Verification items for the finished model (mm, model axes). Coordinates: 2 decimals unless noted, no trailing zeros. Loops run counter-clockwise (first coordinate to the right, second up) from the corner with the lowest first, then second, coordinate; pieces in that order, holes last. Notation, with made-up numbers: (-31.75, 56.5) -> (-14.75, 56.5) arc R21 ccw to (-14.75, 71.5) -> close; hole circle Ø6 at (0, 10). An arc over 180 degrees is marked (long way). Write item = value, one per line.
```python
from build123d import *

# Parameters (mm, degrees)
F1_DEPTH = 3.048


with BuildPart() as f1:
    # F0 (on Front) → F1 (new body)
    with BuildSketch(Plane.XZ):
        with BuildLine():
            Line((9.525, 0), (0, 0))
            Line((0, 0), (0, 9.525))
            ThreePointArc((0, 9.525), (-5.473729162, 7.7951211704), (-8.95924033, 3.2338270994))
            ThreePointArc((-8.95924033, 3.2338270994), (-6.4472498387, -7.0113190283), (3.9721601425, -8.657226392))
            ThreePointArc((3.9721601425, -8.657226392), (8.0174949441, -5.1425090978), (9.525, 0))
        make_face()
        with BuildLine():
            Line((0, 9.525), (0, 0))
            Line((0, 0), (9.525, 0))
            ThreePointArc((9.525, 0), (8.5520017953, 4.1939110974), (5.8317946892, 7.5309890255))
            ThreePointArc((5.8317946892, 7.5309890255), (3.0816354856, 9.0127214388), (0, 9.525))
        make_face()
        with BuildLine():
            ThreePointArc((-8.95924033, 3.2338270994), (-5.473729162, 7.7951211704), (0, 9.525))
            Line((0, 9.525), (0, 47.625))
            ThreePointArc((0, 47.625), (-8.2836905365, 49.957618522), (-14.1330264303, 56.2699800194))
            Line((-14.1330264303, 56.2699800194), (-8.95924033, 3.2338270994))
        make_face()
        with BuildLine():
            Line((0, 47.625), (0, 9.525))
            ThreePointArc((0, 9.525), (3.0816354856, 9.0127214388), (5.8317946892, 7.5309890255))
            Line((5.8317946892, 7.5309890255), (14.4691487973, 56.9685868235))
            ThreePointArc((14.4691487973, 56.9685868235), (8.6118941245, 50.1639246932), (0, 47.625))
        make_face()
        with BuildLine():
            Line((36.5125, 0), (9.525, 0))
            ThreePointArc((9.525, 0), (8.0174949441, -5.1425090978), (3.9721601425, -8.657226392))
            Line((3.9721601425, -8.657226392), (40.3929904428, -6.8223588078))
            ThreePointArc((40.3929904428, -6.8223588078), (37.5504920607, -3.9243721084), (36.5125, 0))
        make_face()
        with BuildLine():
            ThreePointArc((5.8317946892, 7.5309890255), (8.5520017953, 4.1939110974), (9.525, 0))
            Line((9.525, 0), (36.5125, 0))
            ThreePointArc((36.5125, 0), (38.8078464582, 5.5830108061), (44.366360702, 7.9370593243))
            Line((44.366360702, 7.9370593243), (5.8317946892, 7.5309890255))
        make_face()
        with BuildLine():
            ThreePointArc((-14.1330264303, 56.2699800194), (-8.2836905365, 49.957618522), (0, 47.625))
            Line((0, 47.625), (0, 63.5))
            Line((0, 63.5), (0, 79.375))
            ThreePointArc((0, 79.375), (-10.4834895471, 75.4210767935), (-15.7448168762, 65.528883076))
            ThreePointArc((-15.7448168762, 65.528883076), (-15.6397954467, 60.7774233922), (-14.1330264303, 56.2699800194))
        make_face()
        with BuildLine():
            Line((0, 63.5), (0, 47.625))
            ThreePointArc((0, 47.625), (8.6118941245, 50.1639246932), (14.4691487973, 56.9685868235))
            ThreePointArc((14.4691487973, 56.9685868235), (15.5195580181, 60.1594994505), (15.875, 63.5))
            ThreePointArc((15.875, 63.5), (15.5195580181, 66.8405005495), (14.4691487973, 70.0314131765))
            ThreePointArc((14.4691487973, 70.0314131765), (8.6118941245, 76.8360753068), (0, 79.375))
            Line((0, 79.375), (0, 63.5))
        make_face()
        with BuildLine():
            ThreePointArc((44.366360702, 7.9370593243), (38.8078464582, 5.5830108061), (36.5125, 0))
            ThreePointArc((36.5125, 0), (37.5504920607, -3.9243721084), (40.3929904428, -6.8223588078))
            ThreePointArc((40.3929904428, -6.8223588078), (48.3743721084, -6.8995079393), (52.3875, 0))
            ThreePointArc((52.3875, 0), (50.0330108061, 5.6421535418), (44.366360702, 7.9370593243))
        make_face()
        with BuildLine():
            Line((0, 104.775), (0, 79.375))
            ThreePointArc((0, 79.375), (8.6118941245, 76.8360753068), (14.4691487973, 70.0314131765))
            Line((14.4691487973, 70.0314131765), (9.5153598494, 113.8715703832))
            ThreePointArc((9.5153598494, 113.8715703832), (6.581976637, 107.4150011946), (0, 104.775))
        make_face()
        with BuildLine():
            ThreePointArc((-15.7448168762, 65.528883076), (-10.4834895471, 75.4210767935), (0, 79.375))
            Line((0, 79.375), (0, 104.775))
            ThreePointArc((0, 104.775), (-6.581976637, 107.4150011946), (-9.5153598494, 113.8715703832))
            Line((-9.5153598494, 113.8715703832), (-15.7448168762, 65.528883076))
        make_face()
        with BuildLine():
            ThreePointArc((-9.5153598494, 113.8715703832), (-6.581976637, 107.4150011946), (0, 104.775))
            ThreePointArc((0, 104.775), (6.581976637, 107.4150011946), (9.5153598494, 113.8715703832))
            ThreePointArc((9.5153598494, 113.8715703832), (9.5225896574, 114.0857309699), (9.525, 114.3))
            ThreePointArc((9.525, 114.3), (-0.2142690301, 123.8225896574), (-9.5153598494, 113.8715703832))
        make_face()
    extrude(amount=F1_DEPTH)


solid = f1.part
```
1) Sectioned sample at D-D, the plane x = 19. Record the cut outline in (y, z), plus the area to 3 significant figures.
Ans:
outline = (-3.05, -7.9) -> (0, -7.9) -> (0, 7.67) -> (-3.05, 7.67) -> close
area = 47.5 mm2
2) Release check for a two-part mould opening along Z. For faces 1 (the face through (21.928, -1.503, -7.753)), 2 (the face through (-15.65, -1.5, 60.84)), 3 (the face through (10.09, -1.5, 31.9)), 4 (the face through (3, -3.048, 43)) record: pulls with the +Z half, pulls with the -Z half, needs draft (parallel to the pull), parting line crosses it, or undercut.
Ans:
face_1 = pulls with the -Z half
face_2 = parting line crosses it
face_3 = undercut
face_4 = needs draft
3) Sectioned sample at A-A, the plane x = 11.5. Record the cut outline in (y, z), plus the area to 3 significant figures.
Ans:
outline = (-3.05, -8.28) -> (0, -8.28) -> (0, 7.59) -> (-3.05, 7.59) -> close; (-3.05, 39.97) -> (0, 39.97) -> (0, 96.31) -> (-3.05, 96.31) -> close
area = 220 mm2
4) Material ranges on line 1 (Z direction, x = 14.5, y = -1.1); line 2 (X direction, y = -0.95, z = 94); line 3 (X direction, y = -2.7, z = 27.5), recorded low to high.
Ans:
line_1 = -8.13 to 7.62, 57.04 to 69.96
line_2 = -12.08 to 11.76
line_3 = -11.33 to 9.32
5) Depth check by flat-ended pin: pin 1 Ø1.5 at (x, y) = (26, -0.5) entering from -Z. Enter the tip coordinate at first touch or a pass-through.
Ans:
pin_1 = -7.59
6) Sectioned sample at C-C, the plane z = 111. Record the cut outline in (x, y).
Ans:
outline = (-9.89, -3.05) -> (9.84, -3.05) -> (9.84, 0) -> (-9.89, 0) -> close
